```python
from build123d import *

# Parameters (mm, degrees)
SKETCH1_R           = 2.5
BOSS_EXTRUDE1_DEPTH = 2
SKETCH2_W           = 56.957260919
SKETCH2_H           = 2
BOSS_EXTRUDE2_DEPTH = 8
FILLET1_R           = 5


with BuildPart() as part:
    # Sketch1 → Boss-Extrude1 (new body)
    with BuildSketch(Plane(origin=(0, 0, 0), x_dir=(1, 0, 0), z_dir=(0, 1, 0))):
        with BuildLine():
            Line((-18.5, 25.846586538), (-8.5, 25.846586538))
            ThreePointArc((-8.5, 25.846586538), (0, 34.346586538), (8.5, 25.846586538))
            Line((8.5, 25.846586538), (18.457260919, 25.846586538))
            ThreePointArc((18.457260919, 25.846586538), (21.992794825, 24.382120444), (23.457260919, 20.846586538))
            Line((23.457260919, 20.846586538), (23.457260919, 2.336586538))
            ThreePointArc((23.457260919, 2.336586538), (24.921727013, -1.198947367), (28.457260919, -2.663413462))
            Line((28.457260919, -2.663413462), (38.457260919, -2.663413462))
            ThreePointArc((38.457260919, -2.663413462), (41.992794825, -4.127879556), (43.457260919, -7.663413462))
            Line((43.457260919, -7.663413462), (43.457260919, -14.663413462))
            ThreePointArc((43.457260919, -14.663413462), (41.992794825, -18.198947367), (38.457260919, -19.663413462))
            Line((38.457260919, -19.663413462), (23.457260919, -19.663413462))
            Line((23.457260919, -19.663413462), (0, -19.663413462))
            Line((0, -19.663413462), (-18.5, -19.663413462))
            ThreePointArc((-18.5, -19.663413462), (-22.035533906, -18.198947367), (-23.5, -14.663413462))
            Line((-23.5, -14.663413462), (-23.5, 20.846586538))
            ThreePointArc((-23.5, 20.846586538), (-22.035533906, 24.382120444), (-18.5, 25.846586538))
        make_face()
        with Locations((-17, -9.163413462)):
            Circle(SKETCH1_R, mode=Mode.SUBTRACT)
        with Locations((17, -9.163413462)):
            Circle(SKETCH1_R, mode=Mode.SUBTRACT)
        with Locations((0, 25.846586538)):
            Circle(SKETCH1_R, mode=Mode.SUBTRACT)
    extrude(amount=BOSS_EXTRUDE1_DEPTH)

    # Sketch2 → Boss-Extrude2 (add)
    with BuildSketch(Plane(origin=(0, 2, 0), x_dir=(1, 0, 0), z_dir=(0, 1, 0))):
        with Locations((9.978630459, -18.663413462)):
            Rectangle(SKETCH2_W, SKETCH2_H)
    extrude(amount=BOSS_EXTRUDE2_DEPTH)

    # Fillet1
    fillet1_edges = [part.edges().sort_by_distance(p)[0] for p in [
        (-18.5, 10, 18.663413462),
        (38.457260919, 10, 18.663413462),
    ]]
    fillet(fillet1_edges, radius=FILLET1_R)


solid = part.part
```
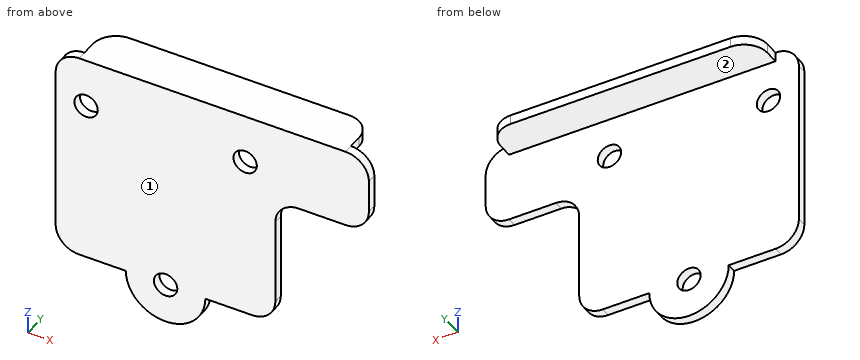
Source: CAD feature listing. Evaluate the final solid. Frame: model axes, mm. Face numbers are marked on the shaded views. A direction names the side the tool comes from. Round coordinates to 2 decimals unless told otherwise and drop trailing zeros. Order: outer loops, then holes, each group sorted by start corner. A loop starts at its lowest first (then second) coordinate and runs counter-clockwise, first axis right, second up. Notation, with made-up numbers: (33.25, 51.5) -> (47.25, 51.5) arc R26 ccw to (47.25, 84.5) -> close; hole circle Ø8 at (19.25, 38.25). An arc over 180 degrees is marked (long way). One line per item, written item: value. Start each with the question number.
Q1. Pin query (flat end, axial travel): pin 1 (1.6 mm diameter, centred on y = 4, z = 19, fed in from +X); pin 2 (3 mm diameter, centred on x = 13, y = 3, fed in from -Z); pin 3 (2.5 mm diameter, centred on x = 7.5, y = 6, fed in from -Z); pin 4 (4.5 mm diameter, centred on x = 17, z = 9.16, fed in from +Y). Return the tip coordinate at first contact, or that it passes through.
Q2. Section query D-D (y = 3.75). Return the cut outline in (x, z), plus the area to 3 significant figures.
Q3. Section query A-A (x = 17). Return the cut outline in (y, z).
Q4. Section query C-C (x = 0). Return the cut outline in (y, z).
Q5. Material intervals for probe 1 along X at (y, z) = (0.75, 9); probe 2 along Z at (x, y) = (0, 1.35); probe 3 along Z at (x, y) = (-14, 0.5), sorted ascending.
Q6. Section query B-B (z = -11). Return the cut outline in (x, y).
Q7. Access query for the marked faces 1 and 2. Directions: +Z, -Z, +X, -X, +Y, -Y. A direction counts if a zero-diameter tool reaches every point of the face in a straight line with its end or side. Return the directions, or none.
Findings below:
1. pin 1: x = 38.46
1. pin 2: z = -25.85
1. pin 3: z = 17.66
1. pin 4: through
2. outline: (-18.5, 17.66) -> (38.46, 17.66) -> (38.46, 19.66) -> (-18.5, 19.66) -> close
2. area: 114 mm²
3. outline: (0, -25.85) -> (2, -25.85) -> (2, 6.66) -> (0, 6.66) -> close; (0, 11.66) -> (2, 11.66) -> (2, 17.66) -> (10, 17.66) -> (10, 19.66) -> (0, 19.66) -> close
4. outline: (0, -34.35) -> (2, -34.35) -> (2, -28.35) -> (0, -28.35) -> close; (0, -23.35) -> (2, -23.35) -> (2, 17.66) -> (10, 17.66) -> (10, 19.66) -> (0, 19.66) -> close
5. probe 1: -23.5 to -19.49, -14.51 to 14.51, 19.49 to 43.46
5. probe 2: -34.35 to -28.35, -23.35 to 19.66
5. probe 3: -25.85 to 19.66
6. outline: (-23.5, 0) -> (23.46, 0) -> (23.46, 2) -> (-23.5, 2) -> close
7. face 1: +Z, -Z, +X, -X, -Y
7. face 2: -Z, +X, -X, +Y
